Here's how the part is built. I have some questions about the finished solid (model axes, mm). Face numbers are marked on the shaded views. A direction names the side the tool comes from. Give positions to 0.01 mm unless a question says otherwise; leave off trailing zeros. Loops run counter-clockwise (first coordinate to the right, second up) from the corner with the lowest first, then second, coordinate; pieces in that order, holes last.
Q1. For the marked faces 1, 2 and 3, which set-ups out of +Z, -Z, +X, -X, +Y, -Y let a thin tool reach every point of the face, with its end or its side?
Q2. If we section it at B-B (y = 7): Please give me the cut outline in (x, z).
Q3. I need wall thicknesses on line 1 (X direction, y = 7.05, z = 8); line 2 (Z direction, x = 0.9, y = 5.25); line 3 (Z direction, x = 0.75, y = 6.75). Which ranges of each line are inside material? Lowest first, please.
Q4. Will these pins go through, and if not, where does the flat tip stop? P1, Ø1.5, axis at x = -0.5, z = 13.5, coming from the +Y side; P2, Ø3, axis at y = 6, z = 13.5, coming from the +X side.
Q5. If we section it at C-C (z = 10.75): Please give me the cut outline in (x, y).
Q6. If we section it at A-A (z = 18.25): Please give me the cut outline in (x, y), plus the area to 3 significant figures.
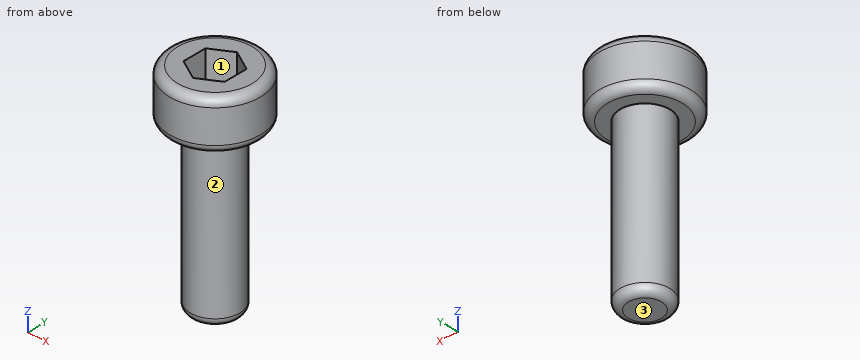
from build123d import *

# Parameters (mm, degrees)
SKETCH011_R     = 2.75
PAD006_DEPTH    = 3
POCKET004_DEPTH = 2
SKETCH013_R     = 1.5
PAD007_DEPTH    = 10
FILLET003_R     = 0.5


with BuildPart() as part:
    # Sketch011 → Pad006 (new body)
    with BuildSketch(Plane.XY):
        Circle(SKETCH011_R)
    extrude(amount=PAD006_DEPTH)

    # Sketch012 (on Face3 of Pad006) → Pocket004 (cut)
    with BuildSketch(Plane.XY.offset(3)):
        Polygon((1.25, -0.721688), (1.25, 0.721688), (0, 1.443376), (-1.25, 0.721688), (-1.25, -0.721688), (0, -1.443376), align=None)
    extrude(amount=-POCKET004_DEPTH, mode=Mode.SUBTRACT)

    # Sketch013 → Pad007 (join)
    with BuildSketch(Plane.XY):
        Circle(SKETCH013_R)
    extrude(amount=-PAD007_DEPTH)

    # Fillet003
    fillet003_edges = [part.edges().sort_by_distance(p)[0] for p in [
        (-2.75, 0, 3),
        (-2.75, 0, 0),
        (-1.5, 0, -10),
    ]]
    fillet(fillet003_edges, radius=FILLET003_R)


with BuildPart() as part_1:
    # Body004 placement: moved
    add(part.part.moved(Location((0, -7, 17))))


with BuildPart() as part_2:
    # Clone placement: moved
    add(part_1.part.moved(Location((0, 14, 0))))


solid = part_2.part
Check sheet entries:
1. face 1: +Z
1. face 2: -Z
1. face 3: -Z, +X, -X, +Y, -Y
2. outline: (-2.75, 17.5) arc R0.5 ccw to (-2.25, 17) - (-1.5, 17) - (-1.5, 7.5) arc R0.5 ccw to (-1, 7) - (1, 7) arc R0.5 ccw to (1.5, 7.5) - (1.5, 17) - (2.25, 17) arc R0.5 ccw to (2.75, 17.5) - (2.75, 19.5) arc R0.5 ccw to (2.25, 20) - (1.25, 20) - (1.25, 18) - (-1.25, 18) - (-1.25, 20) - (-2.25, 20) arc R0.5 ccw to (-2.75, 19.5) - close
3. line 1: x = -1.5 to 1.5
3. line 2: z = 17 to 20
3. line 3: z = 7 to 18
4. P1: stops at y = 8.5
4. P2: stops at x = 1.5
5. outline: circle Ø3 at (0, 7)
6. outline: circle Ø5.5 at (0, 7); hole (-1.25, 6.28) - (0, 5.56) - (1.25, 6.28) - (1.25, 7.72) - (0, 8.44) - (-1.25, 7.72) - close
6. area: 18.3 mm2
